The figure shows three views and two pictorial views of one solid part (mm, origin at its lowest corner). Answer the questions. A direction names the side the tool comes from. Round coordinates to 2 decimals unless told otherwise and drop trailing zeros. Loops run counter-clockwise (first coordinate to the right, second up) from the corner with the lowest first, then second, coordinate; pieces in that order, holes last. Notation, with made-up numbers: (22.5, -26) -> (74.5, -26) arc R33 cw to (74.5, 12) -> close; hole circle Ø9 at (32.5, 4.5). An arc over 180 degrees is marked (long way). Write item = value, one per line. Start each with the question number.
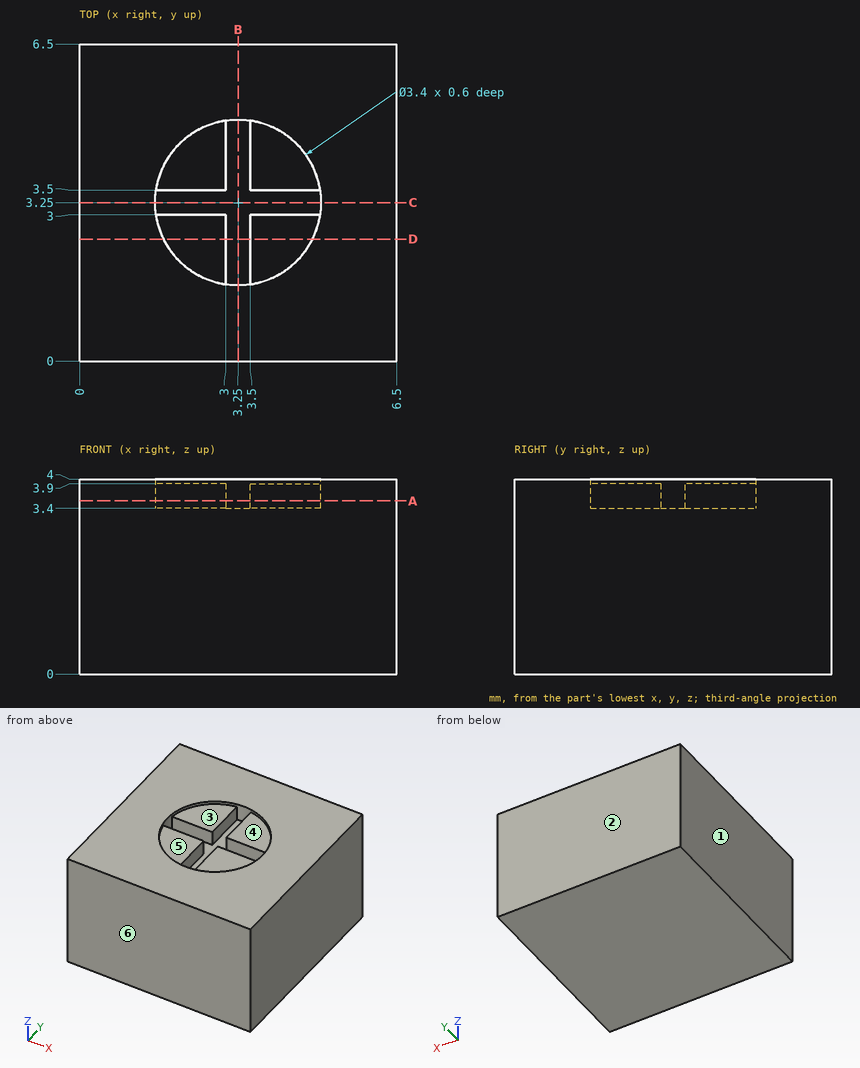
Item 1: Section A-A (z = 3.55) is taken. Determine the outline of the cut face in (x, y), then the cut area to 3 significant figures.
Item 2: Find the intervals of material crossed by line 1 along X through (y, z) = (3.25, 3.65); line 2 along X through (y, z) = (2.75, 3.45), in increasing order. Write a range as [from, to].
Item 3: Section B-B (x = 3.25) is taken. Determine the outline of the cut face in (y, z), then the cut area to 3 significant figures.
Item 4: A flat-ended cylindrical pin translates along its axis: pin 1 (1 mm diameter, centred on x = 3.5, y = 4, fed in from +Z). Find the tip coordinate at first contact, or state that the pin passes through.
Item 5: Section D-D (y = 2.5) is taken. Determine the outline of the cut face in (x, z), then the cut area to 3 significant figures.
Item 6: A tool of negligible diameter and unlimited length cuts with its end or side. For the marked faces 5 and 6, from which of +Z, -Z, +X, -X, +Y, -Y can it reach the whole face along a straight path? Write none if from no direction.
Item 7: The mould has two halves that part along X. Classify the marked faces 1, 2, 3 and 4: pulls with the +X half, pulls with the -X half, needs draft (parallel to the pull), parting line crosses it, or undercut.
Worked answers:
q1.outline = (0, 0) -> (6.5, 0) -> (6.5, 6.5) -> (0, 6.5) -> close; hole (1.57, 3) -> (3, 3) -> (3, 1.57) arc R1.7 ccw to (3.5, 1.57) -> (3.5, 3) -> (4.93, 3) arc R1.7 ccw to (4.93, 3.5) -> (3.5, 3.5) -> (3.5, 4.93) arc R1.7 ccw to (3, 4.93) -> (3, 3.5) -> (1.57, 3.5) arc R1.7 ccw to start
q1.area = 39.1 mm2
q2.line_1 = [0, 1.55], [4.95, 6.5]
q2.line_2 = [0, 3], [3.5, 6.5]
q3.outline = (0, 0) -> (6.5, 0) -> (6.5, 4) -> (4.95, 4) -> (4.95, 3.4) -> (1.55, 3.4) -> (1.55, 4) -> (0, 4) -> close
q3.area = 24.0 mm2
q4.pin_1 = 3.9
q5.outline = (0, 0) -> (6.5, 0) -> (6.5, 4) -> (4.78, 4) -> (4.78, 3.9) -> (3.5, 3.9) -> (3.5, 3.4) -> (3, 3.4) -> (3, 3.9) -> (1.72, 3.9) -> (1.72, 4) -> (0, 4) -> close
q5.area = 25.4 mm2
q6.face_5 = +Z
q6.face_6 = +Z, -Z, +X, -X, -Y
q7.face_1 = pulls with the -X half
q7.face_2 = needs draft
q7.face_3 = undercut
q7.face_4 = undercut
